The listing builds one solid part. Answer for the finished solid, in the listing's coordinates (mm). A direction names the side the tool comes from. Give positions to 0.01 mm unless a question says otherwise; leave off trailing zeros. Write each loop counter-clockwise with the first axis right and the second up, starting at its lowest first coordinate (ties: lowest second). Pieces come first, ordered by that corner, then holes. Notation, with made-up numbers: (37, -36.75) - (79, -36.75) arc R33 ccw to (79, -3.75) - close; hole circle Ø5 at (46.5, 66). An arc over 180 degrees is marked (long way). Return JSON: item names as keys, results as strings.
from build123d import *

# Parameters (mm, degrees)
F0_R          = 10
F1_DEPTH      = 15
F2_DEPTH      = 70
F0_R_2        = 9
F3_DEPTH      = 73
F0_R_3        = 5
F4_DEPTH      = 17
F5_SIZE2      = 9
F5_SIZE       = 9
F7_DEPTH      = 58
F9_DEPTH      = 12.7279220614
F11_DEPTH     = 12.7279220614
F12_T1_DEPTH  = 65.8575805292
F12_T6_DEPTH  = 62.9239144665
F12_T11_DEPTH = 62.9239144665
F12_T14_ANGLE = 91.5672431693
F12_T16_ANGLE = 98.292097676
F12_T18_ANGLE = 98.292097676
F12_T22_DEPTH = 67.925124519
F12_T28_DEPTH = 62.6117965858
F12_T35_DEPTH = 62.6117965858
F12_T42_DEPTH = 67.925124519
F12_T48_DEPTH = 62.6117965858
F12_T55_DEPTH = 62.6117965858


# Not quite as in the source:
# - a fillet or chamfer that OpenCascade refuses, or shapes differently, is made with other operations: its cross-section is extruded or revolved along the edge and cut away or added


with BuildPart() as f1:
    # F0 (on Front) → F1 (new body)
    with BuildSketch(Plane.XZ):
        with BuildLine():
            Line((0, 70), (0, 15))
            Line((0, 15), (27.1394289005, 15))
            ThreePointArc((27.1394289005, 15), (40.3746039083, 43.4577930659), (65, 24))
            ThreePointArc((65, 24), (64.4577930659, 19.3746039083), (62.8605710995, 15))
            Line((62.8605710995, 15), (90, 15))
            Line((90, 15), (90, 70))
            Line((90, 70), (0, 70))
        make_face()
        with Locations((45, 58)):
            Circle(F0_R, mode=Mode.SUBTRACT)
    extrude(amount=F1_DEPTH)

    # F0 (on Front) → F2 (join)
    with BuildSketch(Plane.XZ):
        with BuildLine():
            Line((0, 15), (0, 0))
            Line((0, 0), (90, 0))
            Line((90, 0), (90, 15))
            Line((90, 15), (62.8605710995, 15))
            ThreePointArc((62.8605710995, 15), (45, 4), (27.1394289005, 15))
            Line((27.1394289005, 15), (0, 15))
        make_face()
    extrude(amount=F2_DEPTH)

    # F0 (on Front) → F3 (join)
    with BuildSketch(Plane.XZ):
        with BuildLine():
            ThreePointArc((65, 24), (40.3746039083, 43.4577930659), (27.1394289005, 15))
            ThreePointArc((27.1394289005, 15), (45, 4), (62.8605710995, 15))
            ThreePointArc((62.8605710995, 15), (64.4577930659, 19.3746039083), (65, 24))
        make_face()
        with Locations((45, 24)):
            Circle(F0_R_2, mode=Mode.SUBTRACT)
    extrude(amount=F3_DEPTH)

    # F0 (on Front) → F4 (join)
    with BuildSketch(Plane.XZ):
        with Locations((45, 58)):
            Circle(F0_R)
        with Locations((45, 58)):
            Circle(F0_R_3, mode=Mode.SUBTRACT)
    extrude(amount=F4_DEPTH)

    # F5
    f5_edges = [f1.edges().sort_by_distance(p)[0] for p in [
        (90, -7.5, 70),
        (0, -7.5, 70),
    ]]
    chamfer(f5_edges, length=F5_SIZE, length2=F5_SIZE2)

    # F6 (on face) → F7 (join, through all)
    with BuildSketch(Plane.XZ.offset(15)):
        with BuildLine():
            Line((90, 61), (81, 70))
            Line((81, 70), (53.2287565553, 42.2287565553))
            ThreePointArc((53.2287565553, 42.2287565553), (58.60484202, 38.659750121), (62.5646599663, 33.5646599663))
            Line((62.5646599663, 33.5646599663), (90, 61))
        make_face()
        with BuildLine():
            Line((36.7712434447, 42.2287565553), (9, 70))
            Line((9, 70), (0, 61))
            Line((0, 61), (27.4353400337, 33.5646599663))
            ThreePointArc((27.4353400337, 33.5646599663), (31.39515798, 38.659750121), (36.7712434447, 42.2287565553))
        make_face()
    extrude(amount=F7_DEPTH)

    # F8 (on face) → F9 (cut, through all)
    with BuildSketch(Plane(origin=(5.5, 0, -5.5), x_dir=(0, -1, 0), z_dir=(-0.7071067812, 0, 0.7071067812))):
        Polygon((73, 67.4986548357), (73, 106.7731239592), (15, 106.7731239592), align=None)
    extrude(amount=-F9_DEPTH, mode=Mode.SUBTRACT)

    # F10 (on face) → F11 (cut, through all)
    with BuildSketch(Plane(origin=(39.5, 0, 39.5), x_dir=(0, 1, 0), z_dir=(0.7071067812, 0, 0.7071067812))):
        Polygon((-73, 3.859044529), (-15, 43.1335136524), (-73, 43.1335136524), align=None)
    extrude(amount=-F11_DEPTH, mode=Mode.SUBTRACT)

    # F12: fillet of radius 3 on 9 edges, made by hand

    # F12_s2 → F12_t1 (join)
    with BuildSketch(Plane.XZ.offset(4.1424194708)):
        with BuildLine():
            ThreePointArc((67.2036033112, 15), (64.821605611, 16.1762437234), (64.3074811402, 18.7826086957))
            ThreePointArc((64.3074811402, 18.7826086957), (63.6800176381, 16.8545860133), (62.8605710995, 15))
            Line((62.8605710995, 15), (67.2036033112, 15))
        make_face()
        with BuildLine():
            ThreePointArc((22.7963966888, 15), (25.178394389, 16.1762437234), (25.6925188598, 18.7826086957))
            ThreePointArc((25.6925188598, 18.7826086957), (26.3199823619, 16.8545860133), (27.1394289005, 15))
            Line((27.1394289005, 15), (22.7963966888, 15))
        make_face()
    extrude(amount=F12_T1_DEPTH)


with BuildPart() as f12_tool4:
    # F12_s5 → F12_t6 (new body)
    with BuildSketch(Plane.XZ.offset(10.0760855335)):
        with BuildLine():
            ThreePointArc((35.378550121, 43.621449879), (36.8258280598, 42.8194729683), (38.47814823, 42.9067567153))
            ThreePointArc((38.47814823, 42.9067567153), (37.6169090114, 42.5873604219), (36.7712434447, 42.2287565553))
            Line((36.7712434447, 42.2287565553), (35.378550121, 43.621449879))
        make_face()
    extrude(amount=F12_T6_DEPTH)

    split(bisect_by=Plane(origin=(-25.8358090511, -24.7411221638, 25.8358090511), x_dir=(-0.6916401802, 0.7222422455, 0), z_dir=(0.5855012217, 0.5606929988, -0.5855012217)), keep=Keep.TOP)


with BuildPart() as f1_1:
    add(f1.part)

    # F12_t3: union F12_tool4
    add(f12_tool4.part)


with BuildPart() as f12_tool9:
    # F12_s10 → F12_t11 (new body)
    with BuildSketch(Plane.XZ.offset(10.0760855335)):
        with BuildLine():
            ThreePointArc((51.52185177, 42.9067567153), (53.1741719402, 42.8194729683), (54.621449879, 43.621449879))
            Line((54.621449879, 43.621449879), (53.2287565553, 42.2287565553))
            ThreePointArc((53.2287565553, 42.2287565553), (52.3830909886, 42.5873604219), (51.52185177, 42.9067567153))
        make_face()
    extrude(amount=F12_T11_DEPTH)

    split(bisect_by=Plane(origin=(56.6888603025, -54.2869013815, 56.6888603025), x_dir=(-0.6916401802, -0.7222422455, 0), z_dir=(-0.5855012217, 0.5606929988, -0.5855012217)), keep=Keep.TOP)


with BuildPart() as f1_2:
    add(f1_1.part)

    # F12_t8: union F12_tool9
    add(f12_tool9.part)

    # F12_s13 → F12_t14 (revolve)
    with BuildSketch(Plane(origin=(33.8801327713, 0, 34.8197847954), x_dir=(0, 1, 0), z_dir=(-0.6973700085, 0, -0.7167112886))):
        with BuildLine():
            ThreePointArc((-15, -7.4848722144), (-15.8786796564, -5.3635518709), (-18, -4.4848722144))
            Line((-18, -4.4848722144), (-15, -4.4848722144))
            Line((-15, -4.4848722144), (-15, -7.4848722144))
        make_face()
    revolve(axis=Axis((45, -15, 24), (0, 1, 0)), revolution_arc=F12_T14_ANGLE)

    # F12_s15 → F12_t16 (revolve)
    with BuildSketch(Plane(origin=(14.639534214, 0, -12.2582579265), x_dir=(0, 1, 0), z_dir=(-0.7667085967, 0, 0.6419952708))):
        with BuildLine():
            ThreePointArc((-18, -67.2907935079), (-15.8786796564, -68.1694731643), (-15, -70.2907935079))
            Line((-15, -70.2907935079), (-15, -67.2907935079))
            Line((-15, -67.2907935079), (-18, -67.2907935079))
        make_face()
    revolve(axis=Axis((45, -15, 24), (0, 1, 0)), revolution_arc=F12_T16_ANGLE)

    # F12_s17 → F12_t18 (revolve)
    with BuildSketch(Plane(origin=(13.1100245291, 0, -11.708191847), x_dir=(0, 1, 0), z_dir=(0.7458581541, 0, -0.666104807))):
        with BuildLine():
            ThreePointArc((-15, 24.8753120149), (-15.8786796564, 26.9966323584), (-18, 27.8753120149))
            Line((-18, 27.8753120149), (-15, 27.8753120149))
            Line((-15, 27.8753120149), (-15, 24.8753120149))
        make_face()
    revolve(axis=Axis((45, -15, 24), (0, 1, 0)), revolution_arc=F12_T18_ANGLE)


with BuildPart() as f12_tool20:
    # F12_s21 → F12_t22 (new body)
    with BuildSketch(Plane.XZ.offset(9.6866720668)):
        with BuildLine():
            ThreePointArc((25.9325039488, 35.0674960512), (26.7555146188, 33.5214277242), (26.5749422655, 31.779283224))
            ThreePointArc((26.5749422655, 31.779283224), (26.9830125278, 32.6826356843), (27.4353400337, 33.5646599663))
            Line((27.4353400337, 33.5646599663), (25.9325039488, 35.0674960512))
        make_face()
    extrude(amount=F12_T22_DEPTH)

    split(bisect_by=Plane.XZ.offset(15), keep=Keep.BOTTOM)

    split(bisect_by=Plane(origin=(30.5, 0, 30.5), x_dir=(0, 1, 0), z_dir=(-0.7071067812, 0, -0.7071067812)), keep=Keep.TOP)


with BuildPart() as f1_3:
    add(f1_2.part)

    # F12_t19: union F12_tool20
    add(f12_tool20.part)


with BuildPart() as f12_tool26:
    # F12_s27 → F12_t28 (new body)
    with BuildSketch(Plane.XZ.offset(15)):
        with BuildLine():
            ThreePointArc((25.9325039488, 35.0674960512), (26.7555146188, 33.5214277242), (26.5749422655, 31.779283224))
            ThreePointArc((26.5749422655, 31.779283224), (26.9830125278, 32.6826356843), (27.4353400337, 33.5646599663))
            Line((27.4353400337, 33.5646599663), (25.9325039488, 35.0674960512))
        make_face()
    extrude(amount=F12_T28_DEPTH)

    split(bisect_by=Plane(origin=(-25.8358090511, -24.7411221638, 25.8358090511), x_dir=(-0.6916401802, 0.7222422455, 0), z_dir=(0.5855012217, 0.5606929988, -0.5855012217)), keep=Keep.TOP)

    split(bisect_by=Plane(origin=(30.5, 0, 30.5), x_dir=(0, 1, 0), z_dir=(-0.7071067812, 0, -0.7071067812)), keep=Keep.TOP)

    split(bisect_by=Plane.XZ.offset(73), keep=Keep.BOTTOM)


with BuildPart() as f1_4:
    add(f1_3.part)

    # F12_t25: union F12_tool26
    add(f12_tool26.part)


with BuildPart() as f12_tool33:
    # F12_s34 → F12_t35 (new body)
    with BuildSketch(Plane.XZ.offset(15)):
        with BuildLine():
            ThreePointArc((25.9325039488, 35.0674960512), (26.7555146188, 33.5214277242), (26.5749422655, 31.779283224))
            ThreePointArc((26.5749422655, 31.779283224), (26.9830125278, 32.6826356843), (27.4353400337, 33.5646599663))
            Line((27.4353400337, 33.5646599663), (25.9325039488, 35.0674960512))
        make_face()
    extrude(amount=F12_T35_DEPTH)

    split(bisect_by=Plane(origin=(-25.8358090511, -24.7411221638, 25.8358090511), x_dir=(0.6916401802, -0.7222422455, 0), z_dir=(-0.5855012217, -0.5606929988, 0.5855012217)), keep=Keep.TOP)

    split(bisect_by=Plane(origin=(30.5, 0, 30.5), x_dir=(0, 1, 0), z_dir=(-0.7071067812, 0, -0.7071067812)), keep=Keep.TOP)

    split(bisect_by=Plane.XZ.offset(73), keep=Keep.BOTTOM)


with BuildPart() as f1_5:
    add(f1_4.part)

    # F12_t32: union F12_tool33
    add(f12_tool33.part)


with BuildPart() as f12_tool40:
    # F12_s41 → F12_t42 (new body)
    with BuildSketch(Plane.XZ.offset(9.6866720668)):
        with BuildLine():
            ThreePointArc((63.4250577345, 31.779283224), (63.2444853812, 33.5214277242), (64.0674960512, 35.0674960512))
            Line((64.0674960512, 35.0674960512), (62.5646599663, 33.5646599663))
            ThreePointArc((62.5646599663, 33.5646599663), (63.0169874722, 32.6826356843), (63.4250577345, 31.779283224))
        make_face()
    extrude(amount=F12_T42_DEPTH)

    split(bisect_by=Plane(origin=(14.5, 0, -14.5), x_dir=(0, 1, 0), z_dir=(0.7071067812, 0, -0.7071067812)), keep=Keep.TOP)

    split(bisect_by=Plane.XZ.offset(15), keep=Keep.BOTTOM)


with BuildPart() as f1_6:
    add(f1_5.part)

    # F12_t39: union F12_tool40
    add(f12_tool40.part)


with BuildPart() as f12_tool46:
    # F12_s47 → F12_t48 (new body)
    with BuildSketch(Plane.XZ.offset(15)):
        with BuildLine():
            ThreePointArc((63.4250577345, 31.779283224), (63.2444853812, 33.5214277242), (64.0674960512, 35.0674960512))
            Line((64.0674960512, 35.0674960512), (62.5646599663, 33.5646599663))
            ThreePointArc((62.5646599663, 33.5646599663), (63.0169874722, 32.6826356843), (63.4250577345, 31.779283224))
        make_face()
    extrude(amount=F12_T48_DEPTH)

    split(bisect_by=Plane.XZ.offset(73), keep=Keep.BOTTOM)

    split(bisect_by=Plane(origin=(14.5, 0, -14.5), x_dir=(0, 1, 0), z_dir=(0.7071067812, 0, -0.7071067812)), keep=Keep.TOP)

    split(bisect_by=Plane(origin=(56.6888603025, -54.2869013815, 56.6888603025), x_dir=(-0.6916401802, -0.7222422455, 0), z_dir=(-0.5855012217, 0.5606929988, -0.5855012217)), keep=Keep.TOP)


with BuildPart() as f1_7:
    add(f1_6.part)

    # F12_t45: union F12_tool46
    add(f12_tool46.part)


with BuildPart() as f12_tool53:
    # F12_s54 → F12_t55 (new body)
    with BuildSketch(Plane.XZ.offset(15)):
        with BuildLine():
            ThreePointArc((63.4250577345, 31.779283224), (63.2444853812, 33.5214277242), (64.0674960512, 35.0674960512))
            Line((64.0674960512, 35.0674960512), (62.5646599663, 33.5646599663))
            ThreePointArc((62.5646599663, 33.5646599663), (63.0169874722, 32.6826356843), (63.4250577345, 31.779283224))
        make_face()
    extrude(amount=F12_T55_DEPTH)

    split(bisect_by=Plane.XZ.offset(73), keep=Keep.BOTTOM)

    split(bisect_by=Plane(origin=(14.5, 0, -14.5), x_dir=(0, 1, 0), z_dir=(0.7071067812, 0, -0.7071067812)), keep=Keep.TOP)

    split(bisect_by=Plane(origin=(56.6888603025, -54.2869013815, 56.6888603025), x_dir=(0.6916401802, 0.7222422455, 0), z_dir=(0.5855012217, -0.5606929988, 0.5855012217)), keep=Keep.TOP)


with BuildPart() as f1_8:
    add(f1_7.part)

    # F12_t52: union F12_tool53
    add(f12_tool53.part)


solid = f1_8.part
Item 1: A cutting plane is placed at D-D on x = 19.5. Determine the outline of the cut face in (y, z).
Answer below:
{"outline": "(-70, 0) - (0, 0) - (0, 70) - (-15, 70) - (-15, 59.5) - (-36.93, 59.5) - (-55.73, 41.5) - (-15, 41.5) - (-15, 15) - (-70, 15) - close"}
Item 2: A cutting plane is placed at C-C on y = -36. Determine the outline of the cut face in (x, z).
Answer below:
{"outline": "(0, 0) - (90, 0) - (90, 15) - (67.2, 15) arc R3 cw to (64.31, 18.78) arc R20 ccw to (63.43, 31.78) arc R3 cw to (64.07, 35.07) - (79.94, 50.94) - (70.94, 59.94) - (54.62, 43.62) arc R3 cw to (51.52, 42.91) arc R20 ccw to (38.48, 42.91) arc R3 cw to (35.38, 43.62) - (19.06, 59.94) - (10.06, 50.94) - (25.93, 35.07) arc R3 cw to (26.57, 31.78) arc R20 ccw to (25.69, 18.78) arc R3 cw to (22.8, 15) - (0, 15) - close; hole circle Ø18 at (45, 24)"}
Item 3: The mould has two halves that part along X. Classify faces 6 (the face through (46, -7, 70)), 7 (the face through (90, -19, 10)), 8 (the face through (36.803, -43.709, 42.825)): +X half, -X half, draft (parallel to the pull), parting line (faces both ways), or undercut.
Answer below:
{"face 6": "draft", "face 7": "+X half", "face 8": "undercut"}
Item 4: Flat-ended cylindrical pins translate along their axes: P1, Ø5, axis at y = -51.5, z = 10.5, coming from the -X side; P2, Ø10, axis at x = 40.5, z = 59, coming from the -Y side; P3, Ø7.5, axis at x = 17, z = 41, coming from the -Y side; P4, Ø1.5, axis at y = -41, z = 27, coming from the -X side. Find the tip coordinate at first contact, or state that the pin passes through.
Answer below:
{"P1": "stops at x = 0", "P2": "stops at y = -17", "P3": "stops at y = -58.2", "P4": "stops at x = 25.13"}
Item 5: A cutting plane is placed at B-B on z = 58. Determine the outline of the cut face in (x, y).
Answer below:
{"outline": "(0, -15) - (3, -15) - (3, -21.27) - (21, -40.06) - (21, -15) - (35, -15) - (35, -17) - (40, -17) - (40, 0) - (0, 0) - close; (50, -17) - (55, -17) - (55, -15) - (69, -15) - (69, -40.06) - (87, -21.27) - (87, -15) - (90, -15) - (90, 0) - (50, 0) - close"}
Item 6: For faces 1 (the face through (80, -15, 33)), 2 (the face through (44, -70, 3)), 3 (the face through (44, -15, 69)), 4 (the face through (38.367, -35.989, 30.083)), 5 (the face through (12, -42, 15)), determine the directions among +Z, -Z, +X, -X, +Y, -Y from which every point of the face is accessible in a straight line to the end or side of a thin tool.
Answer below:
{"face 1": "+X, -Y", "face 2": "-Z, -Y", "face 3": "-Y", "face 4": "+Y, -Y", "face 5": "-X, -Y"}
Item 7: Consider L1, parallel to Z at x = 45, y = -6.75; L2, parallel to Z at x = 45, y = -19; L3, parallel to Z at x = 9, y = -52.5. Determine where each line is inside the solid, lowest interval first.
Answer below:
{"L1": "z = 0 to 15, 33 to 53, 63 to 70", "L2": "z = 0 to 15, 33 to 44", "L3": "z = 0 to 15"}
Item 8: A cutting plane is placed at A-A on x = 45. Determine the outline of the cut face in (y, z), then the cut area to 3 significant figures.
Answer below:
{"outline": "(-73, 4) - (-70, 4) - (-70, 0) - (0, 0) - (0, 15) - (-73, 15) - close; (-73, 33) - (0, 33) - (0, 53) - (-17, 53) - (-17, 48) - (-15, 48) - (-15, 47) arc R3 cw to (-18, 44) - (-73, 44) - close; (-17, 63) - (0, 63) - (0, 70) - (-15, 70) - (-15, 68) - (-17, 68) - close", "area": "2,150 mm²"}
